Check sheet for the modelled part. Datum: model origin and axes. Units: mm. A direction names the side the tool comes from. Round coordinates to 2 decimals unless told otherwise and drop trailing zeros. Order: outer loops, then holes, each group sorted by start corner. A loop starts at its lowest first (then second) coordinate and runs counter-clockwise, first axis right, second up.
```python
from build123d import *

# Parameters (mm, degrees)
BOSS_EXTRUDE1_DEPTH = 1.6
SKETCH2_R           = 1.6
CUT_EXTRUDE1_DEPTH  = 1.6


with BuildPart() as part:
    # Sketch1 → Boss-Extrude1 (new body)
    with BuildSketch(Plane(origin=(0, 0, 0), x_dir=(1, 0, 0), z_dir=(0, 1, 0))):
        Polygon((0, 0), (53.3, 0), (53.3, 65), (51.3, 65), (48.3, 68), (16.3, 68), (13.3, 65), (0, 65), align=None)
    extrude(amount=BOSS_EXTRUDE1_DEPTH)

    # Sketch2 → Cut-Extrude1 (cut)
    with BuildSketch(Plane(origin=(0, 1.6, 0), x_dir=(1, 0, 0), z_dir=(0, 1, 0))):
        with Locations(Location((18.3, 65.5, 0), (0, 0, 270))):
            Circle(SKETCH2_R)
        with Locations(Location((46.3, 65.5, 0), (0, 0, 270))):
            Circle(SKETCH2_R)
        with Locations(Location((2.8, 15, 0), (0, 0, 270))):
            Circle(SKETCH2_R)
    extrude(amount=-CUT_EXTRUDE1_DEPTH, mode=Mode.SUBTRACT)


solid = part.part
```
Item 1: Sectioned sample at B-B (y = 0.3). Record the cut outline in (x, z), and give its area (3 significant figures).
Answer:
outline: (0, -65) - (13.3, -65) - (16.3, -68) - (48.3, -68) - (51.3, -65) - (53.3, -65) - (53.3, 0) - (0, 0) - close; hole circle Ø3.2 at (2.8, -15); hole circle Ø3.2 at (18.3, -65.5); hole circle Ø3.2 at (46.3, -65.5)
area: 3,550 mm2
Item 2: Sectioned sample at C-C (x = 46.3). Record the cut outline in (y, z).
Answer:
outline: (0, -68) - (1.6, -68) - (1.6, -67.1) - (0, -67.1) - close; (0, -63.9) - (1.6, -63.9) - (1.6, 0) - (0, 0) - close
Item 3: Access from +Z, -Z, +X, -X, +Y, -Y to the whole of each face (thin tool, end or side, straight path). Record for faces 1 (the cylindrical face through (3.88, 0.81, -16.18)), 2 (the flat face through (52, 1, -65)), 3 (the flat face through (7, 1, -65)).
Answer:
face 1: +Y, -Y
face 2: -Z, +X, +Y, -Y
face 3: -Z, -X, +Y, -Y
Item 4: Release check for a two-part mould opening along X. For faces 4 (the flat face through (0, 1, -33)), 5 (the cylindrical face through (44.88, 0.81, -64.76)), 6 (the flat face through (26, 1.6, -34)), 7 (the flat face through (49.8, 0.8, -66.5)) record: released by +X, released by -X, zero draft, split by the parting line, or undercut.
Answer:
face 4: released by -X
face 5: undercut
face 6: zero draft
face 7: released by +X
Item 5: Sectioned sample at A-A (x = 2.8). Record the cut outline in (y, z).
Answer:
outline: (0, -65) - (1.6, -65) - (1.6, -16.6) - (0, -16.6) - close; (0, -13.4) - (1.6, -13.4) - (1.6, 0) - (0, 0) - close
Item 6: Scan lines: line 1 along X through (y, z) = (0.75, -65.5); line 2 along X through (y, z) = (0.5, -15); line 3 along Z through (x, y) = (18.5, 0.25). Record each from-to range of solid material in increasing order.
Answer:
line 1: x = 13.8 to 16.7, 19.9 to 44.7, 47.9 to 50.8
line 2: x = 0 to 1.2, 4.4 to 53.3
line 3: z = -68 to -67.09, -63.91 to 0
Item 7: Go/stop test with flat-tipped pins: P1, Ø4, axis at x = 2.8, z = -15, coming from the -Y side; P2, Ø3, axis at x = 18.3, z = -65.5, coming from the -Y side. Record where each tip stops, or that it passes through.
Answer:
P1: stops at y = 0
P2: passes through
